Geometry: final body of the model. Coordinates: model frame, mm. Face numbers are marked on the shaded views. A direction names the side the tool comes from. Give positions to 0.01 mm unless a question says otherwise; leave off trailing zeros. Loops run counter-clockwise (first coordinate to the right, second up) from the corner with the lowest first, then second, coordinate; pieces in that order, holes last.
1. Section D-D, the plane y = 20. Output: boundary loops of the cut face in (x, z).
2. Section B-B, the plane y = -4.5. Output: boundary loops of the cut face in (x, z), then the cut area to 3 significant figures.
3. Section C-C, the plane z = 8.5. State how many separate pieces and enclosed holes the cut face has, then the cut area to 3 significant figures.
4. First-contact query: P1, Ø10, axis at x = -24, y = -9.5, coming from the +Z side; P2, Ø12, axis at x = 30, y = 21.5, coming from the +Z side; P3, Ø10, axis at x = -6, y = -26, coming from the +Z side; P4, Ø2.5, axis at x = -1, y = 31.5, coming from the +Z side. Flat tips, straight axial feed; report the tip coordinate or a pass-through.
5. Access query for the marked faces 1, 2 and 3. Directions: +Z, -Z, +X, -X, +Y, -Y. A direction counts if a zero-diameter tool reaches every point of the face in a straight line with its end or side. Return the directions, or none.
6. Section A-A, the plane y = 31. Output: boundary loops of the cut face in (x, z), then the cut area to 3 significant figures.
7. Material intervals for line 1 along X through (y, z) = (0, 8); line 2 along X through (y, z) = (20, 2.25); line 3 along X through (y, z) = (26.5, 16.5), sorted ascending.
8. Draft query along Y for the marked faces 4, 5, 6 and 7. Return one class per face: +Y half, -Y half, draft (parallel to the pull), parting line (faces both ways), or undercut.
Autodesk Inventor part; units mm, degrees
ref_plane "YZ Plane" through (0, 0, 0) normal (1, 0, 0) x (0, 1, 0)
ref_plane "XZ Plane" through (0, 0, 0) normal (0, 1, 0) x (-1, 0, 0)
ref_plane "XY Plane" through (0, 0, 0) normal (0, 0, 1) x (1, 0, 0)
sketch "Sketch1" plane through (0, 0, 0) normal (0, 0, 1) x (1, 0, 0)
  line L0 (-40, -40) -> (40, -40)
  line L1 (40, -40) -> (40, 40)
  line L2 (40, 40) -> (-40, 40)
  line L3 (-40, 40) -> (-40, -40)
  line L4 (-40, -40) -> (40, 40) construction
  line L5 (40, -40) -> (-40, 40) construction
  circle A0 centre (0, 0) radius 37
  dimension "d0" = 80
  dimension "d1" = 80
  dimension "d2" = 74
extrude "Extrusion1" add sketch "Sketch1" along normal blind 25
sketch "Sketch2" plane through (0, 0, 25) normal (0, 0, 1) x (1, 0, 0)
  line L0 (-35.75, -35.75) -> (35.75, -35.75) construction
  line L1 (35.75, -35.75) -> (35.75, 35.75) construction
  line L2 (35.75, 35.75) -> (-35.75, 35.75) construction
  line L3 (-35.75, 35.75) -> (-35.75, -35.75) construction
  line L4 (-35.75, -35.75) -> (35.75, 35.75) construction
  line L5 (35.75, -35.75) -> (-35.75, 35.75) construction
  point P0 (0, 0)
  dimension "d5" = 71.5
  dimension "d6" = 71.5
hole "Hole1" at (-35.75, 35.75, 25) at (-35.75, -35.75, 25) at (35.75, -35.75, 25) at (35.75, 35.75, 25) direction (0, 0, -1) diameter 4.5 end through all
sketch "Sketch3" plane through (0, 0, 0) normal (0, 0, -1) x (-1, 0, 0)
  line L0 (40, -40) -> (-40, -40)
  line L1 (-2.5, -40) -> (2.5, -40)
  line L2 (2.5, -40) -> (2.5, -2.5)
  line L3 (2.5, -2.5) -> (40, -2.5)
  line L4 (40, 40) -> (40, -40)
  line L5 (40, -2.5) -> (40, 2.5)
  line L6 (40, 2.5) -> (2.5, 2.5)
  line L7 (2.5, 2.5) -> (2.5, 40)
  line L8 (2.5, 40) -> (-2.5, 40)
  line L9 (-2.5, 40) -> (-2.5, 2.5)
  line L10 (-2.5, 2.5) -> (-40, 2.5)
  line L11 (-40, 2.5) -> (-40, -2.5)
  line L12 (-40, -40) -> (-40, 40)
  line L13 (-40, -2.5) -> (-2.5, -2.5)
  line L14 (-2.5, -40) -> (-2.5, -2.5)
  point P0 (0, 0)
  point P1 (-40, 0)
  point P2 (40, 0)
  point P3 (0, -40)
  point P4 (0, 40)
  dimension "d14" = 5
  dimension "d15" = 5
extrude "Extrusion2" add sketch "Sketch3" against normal blind 3 contours L0 L14 L13 L11 L10 L9 L8 L7 L6 L4 L3 L2
sketch "Sketch4" plane through (0, 0, 3) normal (0, 0, 1) x (1, 0, 0)
  circle A0 centre (0, 0) radius 16.5
  dimension "d18" = 33
extrude "Extrusion3" add sketch "Sketch4" along normal blind 20
sketch "Sketch5" plane through (0, 0, 0) normal (1, 0, 0) x (0, 1, 0)
  line L0 (9.7071, 5.4142) -> (-6.8787, 22)
  line L1 (-6.8787, 22) -> (-8.2929, 20.5858)
  line L2 (-8.2929, 20.5858) -> (8.2929, 4)
  line L3 (8.2929, 4) -> (9.7071, 5.4142)
  line L4 (16.3095, 3) -> (36.9154, 3)
  line L5 (16.5, 23) -> (-16.5, 23)
  point P0 (0, 0)
  point P1 (0, 12.2929)
  dimension "d21" = 1
  dimension "d22" = 1
  dimension "d23" = 2
  dimension "d24" = 45
extrude "Extrusion4" add sketch "Sketch5" along normal blind 35
fillet "Fillet1" radius 2 2 edges at (35, -7.5858, 21.2929) (35, 9, 4.7071)
pattern_circular "Circular Pattern2" count 6 over 360 about axis through (0, 0, -10) along (0, 0, 1) of "Extrusion4", "Fillet1"
fillet "Fillet2" radius 4 4 edges at (40, -40, 12.5) (-40, -40, 12.5) (-40, 40, 12.5) (40, 40, 12.5)
properties part number "Lüfter"
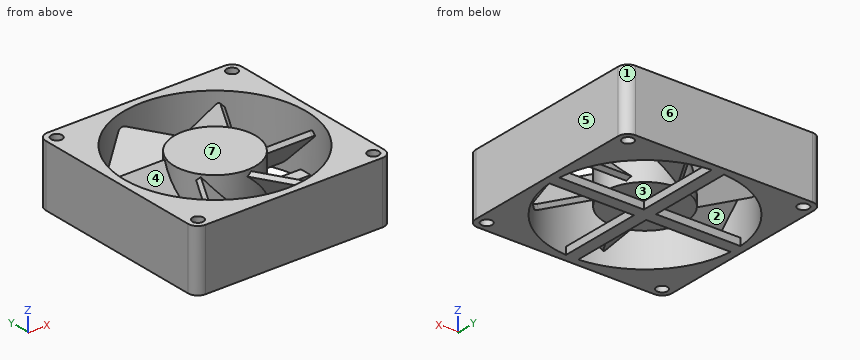
Answers below:
1. outline: (-40, 0) - (-31.13, 0) - (-31.13, 25) - (-40, 25) - close; (-22.76, 5.41) - (-21.12, 4) - (-1.97, 20.59) - (-3.6, 22) - close; (-2.5, 0) - (2.5, 0) - (2.5, 3) - (-2.5, 3) - close; (0.34, 5.41) - (1.97, 4) - (21.12, 20.59) - (19.49, 22) - close; (31.13, 0) - (40, 0) - (40, 25) - (31.13, 25) - close
2. outline: (-40, 0) - (-36.73, 0) - (-36.73, 25) - (-40, 25) - close; (-35, 7.79) - (-15.87, 7.79) - (-15.87, 3) - (-2.5, 3) - (-2.5, 0) - (2.5, 0) - (2.5, 3) - (15.87, 3) - (15.87, 16.79) - (35, 16.79) - (35, 19.62) - (15.87, 19.62) - (15.87, 23) - (-15.87, 23) - (-15.87, 10.62) - (-35, 10.62) - close; (36.73, 0) - (40, 0) - (40, 25) - (36.73, 25) - close
2. area: 922 mm2
3. separate pieces: 2
3. enclosed holes: 5
3. area: 3,210 mm2
4. P1: stops at z = 10.62
4. P2: stops at z = 25
4. P3: stops at z = 12.32
4. P4: stops at z = 3
5. face 1: +Z, -Z, +X, +Y
5. face 2: none
5. face 3: -Z
6. outline: (-40, 0) - (-20.2, 0) - (-20.2, 25) - (-40, 25) - close; (-16.31, 13.67) - (-8.32, 20.59) - (-9.96, 22) - (-16.31, 16.5) - close; (-2.5, 0) - (2.5, 0) - (2.5, 3) - (-2.5, 3) - close; (6.69, 5.41) - (8.32, 4) - (16.31, 10.91) - (16.31, 13.74) - close; (20.2, 0) - (40, 0) - (40, 25) - (20.2, 25) - close
6. area: 1,050 mm2
7. line 1: x = -40 to -37, -16.5 to 16.5, 37 to 40
7. line 2: x = -40 to -31.13, -2.5 to 2.5, 31.13 to 40
7. line 3: x = -40 to -25.82, -13.71 to -10.44, 16.89 to 20.16, 25.82 to 40
8. face 4: undercut
8. face 5: draft
8. face 6: +Y half
8. face 7: undercut
